from build123d import *

# Parameters (mm, degrees)
F0_R     = 12.49
F1_DEPTH = 2.84
F2_R     = 8.99
F3_DEPTH = 0.12
F4_R     = 11.08
F5_DEPTH = 26.56
F6_R     = 6.4
F7_DEPTH = 29.56


with BuildPart() as f1:
    # F0 (on Right) → F1 (new body)
    with BuildSketch(Plane.YZ):
        Circle(F0_R)
    extrude(amount=F1_DEPTH)

    # F2 (on Right) → F3 (join)
    with BuildSketch(Plane.YZ):
        Circle(F2_R)
    extrude(amount=-F3_DEPTH)

    # F4 (on face) → F5 (join)
    with BuildSketch(Plane(origin=(-0.12, 0, 0), x_dir=(0, -1, 0), z_dir=(-1, 0, 0))):
        Circle(F4_R)
    extrude(amount=F5_DEPTH)

    # F6 (on face) → F7 (cut)
    with BuildSketch(Plane.YZ.offset(2.84)):
        Circle(F6_R)
    extrude(amount=-F7_DEPTH, mode=Mode.SUBTRACT)


solid = f1.part
Input: part model. Units: mm. Frame: model coordinates. Coordinates: 2 decimals unless noted, no trailing zeros. Loops run counter-clockwise (first coordinate to the right, second up) from the corner with the lowest first, then second, coordinate; pieces in that order, holes last.
Q1. Cut plane A-A (y = 0). Output: boundary loops of the cut face in (x, z), then the cut area to 3 significant figures.
Q2. Cut plane D-D (z = 10.5). Output: boundary loops of the cut face in (x, y), then the cut area to 3 significant figures.
Q3. Contact query for flat-ended pins moving along their axis: pin 1 (10 mm diameter, centred on x = -11.5, y = -5, fed in from +Z); pin 2 (12 mm diameter, centred on x = -18, z = -10, fed in from -Y); pin 3 (1.5 mm diameter, centred on x = -5, z = -4.5, fed in from -Y); pin 4 (7.5 mm diameter, centred on y = 0, z = 0, fed in from +X). Output: stop coordinate, or through.
Q4. Cut plane C-C (x = -1.75). Output: boundary loops of the cut face in (y, z), then the cut area to 3 significant figures.
Q5. Material intervals for line 1 (Z direction, x = -7.75, y = 0); line 2 (X direction, y = 11, z = 5); line 3 (Y direction, x = -6.5, z = -2.25), sorted ascending.
Q6. Draft query along Z for faces 1 (the face through (-13.214, -10.568, 3.328)), 2 (the face through (-26.68, -5, -5)), 3 (the face through (-11.71, -5.08, -3.89)). Return one class per face: +Z half, -Z half, draft (parallel to the pull), parting line (faces both ways), or undercut.
Working result:
1. outline: (-26.68, -11.08) - (-0.12, -11.08) - (-0.12, -8.99) - (0, -8.99) - (0, -12.49) - (2.84, -12.49) - (2.84, -6.4) - (-26.68, -6.4) - close; (-26.68, 6.4) - (2.84, 6.4) - (2.84, 12.49) - (0, 12.49) - (0, 8.99) - (-0.12, 8.99) - (-0.12, 11.08) - (-26.68, 11.08) - close
1. area: 284 mm2
2. outline: (-26.68, -3.54) - (-0.12, -3.54) - (-0.12, 3.54) - (-26.68, 3.54) - close; (0, -6.76) - (2.84, -6.76) - (2.84, 6.76) - (0, 6.76) - close
2. area: 226 mm2
3. pin 1: stops at z = 11.08
3. pin 2: stops at y = -10.33
3. pin 3: stops at y = -10.43
3. pin 4: passes through
4. outline: circle Ø22.16 at (0, 0); hole circle Ø12.8 at (0, 0)
4. area: 257 mm2
5. line 1: z = -11.08 to -6.4, 6.4 to 11.08
5. line 2: x = 0 to 2.84
5. line 3: y = -10.85 to -5.99, 5.99 to 10.85
6. face 1: parting line
6. face 2: draft
6. face 3: undercut
